Geometry check sheet. Reference: the model listing, model coordinates, mm. Face numbers are marked on the shaded views. A direction names the side the tool comes from. Give positions to 0.01 mm unless a question says otherwise; leave off trailing zeros. Order: outer loops, then holes, each group sorted by start corner. A loop starts at its lowest first (then second) coordinate and runs counter-clockwise, first axis right, second up. Notation, with made-up numbers: M 65.25,29.25 L 98.25,29.25 A18 cw 98.25,61.25 Z; hole C 54,-14 d8. An arc over 180 degrees is marked long. Put each result on its own line as item: value. Start each with the question number.
Q1. Access from +Z, -Z, +X, -X, +Y, -Y to the whole of each face (thin tool, end or side, straight path). Record for the marked faces 1 and 2.
Q2. Go/stop test with flat-tipped pins: pin 1 (1.5 mm diameter, centred on x = -1.5, y = 1, fed in from -Z); pin 2 (3 mm diameter, centred on x = 0, z = 2, fed in from -Y); pin 3 (2 mm diameter, centred on y = 2, z = 5.5, fed in from -X). Record where each tip stops, or that it passes through.
Q3. Material ranges on L1, parallel to Z at x = -1.1, y = -1.75; L2, parallel to Y at x = -1.3, z = 11.5; L3, parallel to Y at x = -0.5, z = 5.5, recorded low to high.
Q4. Section check A-A on z = 8. Record the cut outline in (x, y), then the cut area to 3 significant figures.
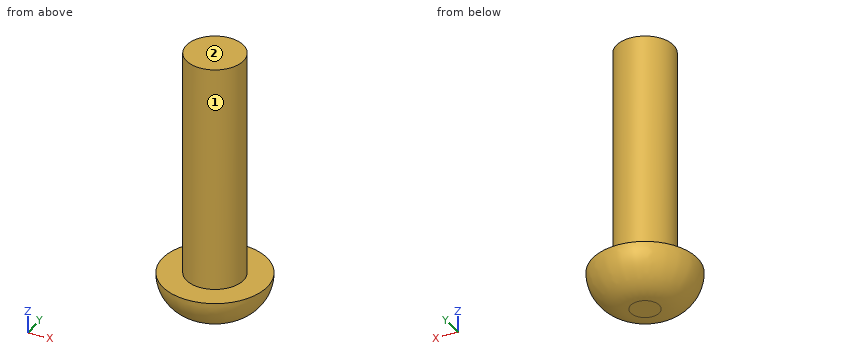
Autodesk Inventor part; units mm, degrees
ref_plane "YZ Plane" through (0, 0, 0) normal (1, 0, 0) x (0, 1, 0)
ref_plane "XZ Plane" through (0, 0, 0) normal (0, 1, 0) x (-1, 0, 0)
ref_plane "XY Plane" through (0, 0, 0) normal (0, 0, 1) x (1, 0, 0)
sketch "スケッチ1" plane through (0, 0, 0) normal (0, 0, 1) x (1, 0, 0)
  circle A0 centre (0, 0) radius 1.5
  dimension "d0" = 3
extrude "押し出し1" add sketch "スケッチ1" along normal blind 12
sketch "スケッチ2" plane through (0, 0, 0) normal (0, 0, -1) x (-1, 0, 0)
  circle A0 centre (0, 0) radius 2.75
  dimension "d3" = 5.5
extrude "押し出し2" add sketch "スケッチ2" along normal blind 2
fillet "フィレット1" radius 2 1 edges at (2.75, 0, -2)
thread "ねじ1"
properties part number "ネジ鍋m3,12" material "鋼、高強度、低合金"
Results found:
1. face 1: +Z
1. face 2: +Z, +X, -X, +Y, -Y
2. pin 1: stops at z = -1.98
2. pin 2: stops at y = -1.5
2. pin 3: stops at x = -1.12
3. L1: z = -1.51 to 0
3. L2: y = -0.75 to 0.75
3. L3: y = -1.41 to 1.41
4. outline: C 0,0 d3
4. area: 7.07 mm^2
